Build history of the part. All positions in model axes, mm. Round coordinates to 2 decimals unless told otherwise and drop trailing zeros. Write each loop counter-clockwise with the first axis right and the second up, starting at its lowest first coordinate (ties: lowest second). Pieces come first, ordered by that corner, then holes. Notation, with made-up numbers: M -10,45 L 7,45 A19 cw 7,54 Z; hole C 59,47.25 d3. An arc over 180 degrees is marked long. Write item = value, one per line.
from build123d import *

# Parameters (mm, degrees)
F1_DEPTH = 5
F2_SIZE  = 5
F3_W     = 10
F3_H     = 5
F4_DEPTH = 5


# Not quite as in the source:
# - a pattern or mirror of a feature is missing from the dataset's text; its kind, count and spacing are read off the source's solid


with BuildPart() as f1:
    # F0 (on Front) → F1 (new body)
    with BuildSketch(Plane.XZ):
        Polygon((-26.5, 32.125), (-50, 32.125), (-50, -32.125), (-26.5, -32.125), (-26.5, -24.125), (-28, -24.125), (-28, -21.125), (-26.5, -21.125), (-26.5, -19.125), (-25, -19.125), (-23.5, -19.125), (-23.5, -21.125), (-22, -21.125), (-22, -24.125), (-23.5, -24.125), (-23.5, -32.125), (-1.5, -32.125), (-1.5, -24.125), (-3, -24.125), (-3, -21.125), (-1.5, -21.125), (-1.5, -19.125), (0, -19.125), (1.5, -19.125), (1.5, -21.125), (3, -21.125), (3, -24.125), (1.5, -24.125), (1.5, -32.125), (23.5, -32.125), (23.5, -24.125), (22, -24.125), (22, -21.125), (23.5, -21.125), (23.5, -19.125), (25, -19.125), (26.5, -19.125), (26.5, -21.125), (28, -21.125), (28, -24.125), (26.5, -24.125), (26.5, -32.125), (50, -32.125), (50, 32.125), (26.5, 32.125), (26.5, 24.125), (28, 24.125), (28, 21.125), (26.5, 21.125), (26.5, 19.125), (25, 19.125), (23.5, 19.125), (23.5, 21.125), (22, 21.125), (22, 24.125), (23.5, 24.125), (23.5, 32.125), (1.5, 32.125), (1.5, 24.125), (3, 24.125), (3, 21.125), (1.5, 21.125), (1.5, 19.125), (0, 19.125), (-1.5, 19.125), (-1.5, 21.125), (-3, 21.125), (-3, 24.125), (-1.5, 24.125), (-1.5, 32.125), (-23.5, 32.125), (-23.5, 24.125), (-22, 24.125), (-22, 21.125), (-23.5, 21.125), (-23.5, 19.125), (-25, 19.125), (-26.5, 19.125), (-26.5, 21.125), (-28, 21.125), (-28, 24.125), (-26.5, 24.125), align=None)
        with BuildLine():
            Line((15, -12.5), (-15, -12.5))
            ThreePointArc((-15, -12.5), (-27.5, 0), (-15, 12.5))
            Line((-15, 12.5), (15, 12.5))
            ThreePointArc((15, 12.5), (27.5, 0), (15, -12.5))
        make_face(mode=Mode.SUBTRACT)
        Polygon((1.5, 32.125), (-1.5, 32.125), (-1.5, 24.125), (-3, 24.125), (-3, 21.125), (-1.5, 21.125), (-1.5, 19.125), (0, 19.125), (1.5, 19.125), (1.5, 21.125), (3, 21.125), (3, 24.125), (1.5, 24.125), align=None)
        Polygon((-1.5, -24.125), (-1.5, -32.125), (1.5, -32.125), (1.5, -24.125), (3, -24.125), (3, -21.125), (1.5, -21.125), (1.5, -19.125), (0, -19.125), (-1.5, -19.125), (-1.5, -21.125), (-3, -21.125), (-3, -24.125), align=None)
    extrude(amount=F1_DEPTH)

    # F2
    f2_edges = [f1.edges().sort_by_distance(p)[0] for p in [
        (-50, -2.5, 32.125),
        (50, -2.5, 32.125),
        (-50, -2.5, -32.125),
        (50, -2.5, -32.125),
    ]]
    chamfer(f2_edges, length=F2_SIZE)

    # F3 (on face) → F4 (join)
    with BuildSketch(Plane(origin=(0, 0, -32.125), x_dir=(1, 0, 0), z_dir=(0, 0, -1))):
        with Locations((35, 2.5)):
            Rectangle(F3_W, F3_H)
        with Locations((15, 2.5)):
            Rectangle(F3_W, F3_H)
        with Locations((-15, 2.5)):
            Rectangle(F3_W, F3_H)
        with Locations((-35, 2.5)):
            Rectangle(F3_W, F3_H)
    f4 = extrude(amount=F4_DEPTH)

    # F4_copies: F4 across plane
    add(f4.mirror(Plane.XY))


solid = f1.part
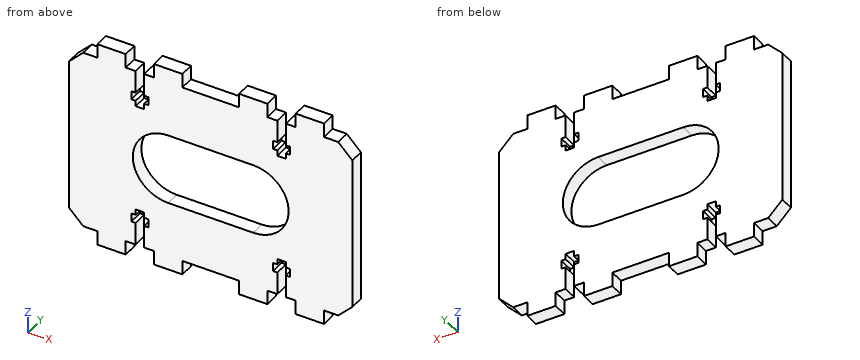
1. Band-saw the part on A-A (z = 22.5). List the corners of the cut face in (x, y).
Responses:
outline = M -50,-5 L -28,-5 L -28,0 L -50,0 Z; M -22,-5 L 22,-5 L 22,0 L -22,0 Z; M 28,-5 L 50,-5 L 50,0 L 28,0 Z
2. Band-saw the part on C-C (x = 17.5). List the corners of the cut face in (y, z) (3 decimals), plus the area to 3 significant figures.
Responses:
outline = M -5,-37.125 L 0,-37.125 L 0,-12.247 L -5,-12.247 Z; M -5,12.247 L 0,12.247 L 0,37.125 L -5,37.125 Z
area = 249 mm²
3. Probe probe 1 along X at (y, z) = (-2.55, 26); probe 2 along Z at (x, y) = (14.5, -0.2) (3 decimals); probe 3 along X at (y, z) = (-2.4, 34.5). List the from-to ranges inside material, lowest first.
Responses:
probe_1 = -50 to -26.5, -23.5 to 23.5, 26.5 to 50
probe_2 = -37.125 to -12.5, 12.5 to 37.125
probe_3 = -40 to -30, -20 to -10, 10 to 20, 30 to 40
4. Flat gauge pins, fed straight in: pin 1 (1.5 mm diameter, centred on x = 29, y = -4, fed in from -Z) (3 decimals); pin 2 (1.8 mm diameter, centred on x = 21.5, y = -2.5, fed in from +Z) (3 decimals). Where does each tip first touch, or does it go through?
Responses:
pin_1 = -32.125
pin_2 = 32.125
5. Band-saw the part on B-B (z = 0). List the corners of the cut face in (x, y).
Responses:
outline = M -50,-5 L -27.5,-5 L -27.5,0 L -50,0 Z; M 27.5,-5 L 50,-5 L 50,0 L 27.5,0 Z
